```python
from build123d import *

# Parameters (mm, degrees)
SKETCH1_R               = 55.585
SKETCH1_R_2             = 17
BOSS_EXTRUDE1_DEPTH     = 10
SKETCH2_W               = 29.3
SKETCH2_H               = 36
SKETCH2_W_2             = 25.2
SKETCH2_H_2             = 32.5
BOSS_EXTRUDE2_DEPTH     = 8.5
CUT_EXTRUDE1_DEPTH      = 10
CUT_EXTRUDE1_DEPTH_BACK = 10
SKETCH4_R               = 12.75
CUT_EXTRUDE2_START      = 10
SKETCH5_R               = 17
CUT_EXTRUDE2_DEPTH      = 10
SKETCH6_R               = 5
CUT_EXTRUDE3_DEPTH      = 10
SKETCH8_R               = 5
SKETCH8_W               = 16
SKETCH8_H               = 3
CUT_EXTRUDE4_DEPTH      = 10


with BuildPart() as part:
    # Sketch1 → Boss-Extrude1 (new body)
    with BuildSketch(Plane(origin=(0, 0, 0), x_dir=(1, 0, 0), z_dir=(0, 1, 0))):
        with Locations(Location((0, 0, 0), (0, 0, 270))):
            Circle(SKETCH1_R)
        with Locations(Location((0, 0, 0), (0, 0, 270))):
            Circle(SKETCH1_R_2, mode=Mode.SUBTRACT)
    extrude(amount=-BOSS_EXTRUDE1_DEPTH)

    # Sketch2 → Boss-Extrude2 (add)
    with BuildSketch(Plane(origin=(0, 0, 0), x_dir=(1, 0, 0), z_dir=(0, 1, 0))):
        with Locations((16, -25)):
            Rectangle(SKETCH2_W, SKETCH2_H)
        with Locations((16, -25)):
            Rectangle(SKETCH2_W_2, SKETCH2_H_2, mode=Mode.SUBTRACT)
    extrude(amount=BOSS_EXTRUDE2_DEPTH)

    # Sketch4 → Cut-Extrude1 (cut, two sides: drawn at the far end of the back side and taken through both)
    with BuildSketch(Plane(origin=(0, 0, 0), x_dir=(1, 0, 0), z_dir=(0, 1, 0)).offset(-CUT_EXTRUDE1_DEPTH_BACK)):
        with Locations(Location((19.6, -28.5, 0), (0, 0, 270))):
            Circle(SKETCH4_R)
    extrude(amount=CUT_EXTRUDE1_DEPTH + CUT_EXTRUDE1_DEPTH_BACK, mode=Mode.SUBTRACT)

    # Sketch5 → Cut-Extrude2 (cut)
    with BuildSketch(Plane(origin=(0, 0, 0), x_dir=(1, 0, 0), z_dir=(0, 1, 0)).offset(CUT_EXTRUDE2_START)):
        with Locations(Location((0, 0, 0), (0, 0, 270))):
            Circle(SKETCH5_R)
    extrude(amount=-CUT_EXTRUDE2_DEPTH, mode=Mode.SUBTRACT)

    # Sketch6 → Cut-Extrude3 (cut)
    with BuildSketch(Plane(origin=(0, 0, 0), x_dir=(1, 0, 0), z_dir=(0, 1, 0))):
        with Locations(Location((42.877793379, -13.088165395, 0), (0, 0, 270))):
            Circle(SKETCH6_R)
    extrude(amount=-CUT_EXTRUDE3_DEPTH, mode=Mode.SUBTRACT)

    # Sketch8 → Cut-Extrude4 (cut)
    with BuildSketch(Plane(origin=(0, 0, 0), x_dir=(1, 0, 0), z_dir=(0, 1, 0))):
        with Locations(Location((-22.482738101, 29, 0), (0, 0, 270))):
            Circle(SKETCH8_R)
        with Locations((0, 27.5)):
            Rectangle(SKETCH8_W, SKETCH8_H)
    extrude(amount=-CUT_EXTRUDE4_DEPTH, mode=Mode.SUBTRACT)


solid = part.part
```
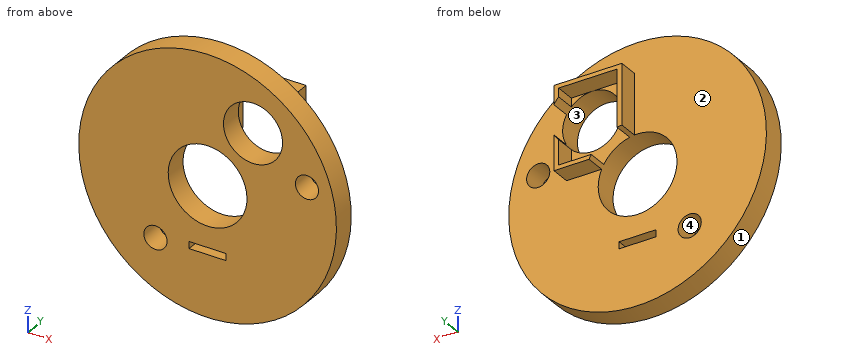
Can you work these out from the model? Positions are in its coordinate system, mm. Face numbers are marked on the shaded views. Round coordinates to 2 decimals unless told otherwise and drop trailing zeros. Loops run counter-clockwise (first coordinate to the right, second up) from the corner with the lowest first, then second, coordinate; pieces in that order, holes last. Notation, with made-up numbers: M -21.5,45.5 L 6.5,45.5 A16 ccw 6.5,51.5 Z; hole C 74.25,9.5 d8. An arc over 180 degrees is marked long. Write item = value, one per line. Start each with the question number.
(1) If we mould it in two halves opening along Z, with no side actions, what happens to the marked faces 1, 2, 3 and 4? For each: released by +Z, released by -Z, zero draft, split by the parting line, or undercut.
(2) Suppose I cut it at C-C on x = 22. Write out the boundary of the cut face in (y, z).
(3) I'm going to push flat-ended pins straight in: P1, Ø4, axis at x = 13, y = 5, coming from the -Z side; P2, Ø2.5, axis at y = 4, z = 14, coming from the +X side; P3, Ø4, axis at x = 18.5, y = 2.5, coming from the +Z side; P4, Ø16, axis at x = -22.48, z = -29, coming from the -Y side. Where does each tip first touch, or does it pass through?
(4) Suppose I cut it at B-B on z = 0. Write out the boundary of the cut face in (x, y) (3 decimals).
(5) Suppose I cut it at D-D on z = -12. Write out the boundary of the cut face in (x, y).
(6) Suppose I cut it at A-A on x = 0. Write out the boundary of the cut face in (y, z) (3 decimals).
(7) I need wall thicknesses on line 1 along Z through (x, y) = (1, -7.5); line 2 along X through (y, z) = (5.75, 40); line 3 along Z through (x, y) = (3, -2.5). Which ranges of each line are inside material? Lowest first, please.
Answer block:
q1.face_1 = split by the parting line
q1.face_2 = zero draft
q1.face_3 = undercut
q1.face_4 = undercut
q2.outline = M -10,-51.05 L 0,-51.05 L 0,7 L 8.5,7 L 8.5,8.75 L 0,8.75 L 0,15.98 L -10,15.98 Z; M -10,41.02 L 0,41.02 L 0,41.25 L 8.5,41.25 L 8.5,43 L 0,43 L 0,51.05 L -10,51.05 Z
q3.P1 = 8
q3.P2 = 30.65
q3.P3 = 43
q3.P4 = -10
q4.outline = M -55.585,-10 L -17,-10 L -17,0 L -55.585,0 Z; M 17,-10 L 55.585,-10 L 55.585,0 L 17,0 Z
q5.outline = M -54.27,-10 L -12.04,-10 L -12.04,0 L -54.27,0 Z; M 12.04,-10 L 54.27,-10 L 54.27,0 L 12.04,0 Z
q6.outline = M -10,-55.585 L 0,-55.585 L 0,-29 L -10,-29 Z; M -10,-26 L 0,-26 L 0,-17 L -10,-17 Z; M -10,17 L 0,17 L 0,55.585 L -10,55.585 Z
q7.line_1 = -55.58 to -29, -26 to -16.97, 16.97 to 55.58
q7.line_2 = 1.35 to 3.4, 28.6 to 30.65
q7.line_3 = -55.5 to -29, -26 to -16.73, 16.73 to 55.5
